from build123d import *

# Parameters (mm, degrees)
SKETCH_1_R          = 30
EXTRUDE_1_DEPTH     = 98
SKETCH_2_R          = 17.5
CUT_EXTRUDE_1_DEPTH = 25
SKETCH_3_R          = 12.5
CUT_EXTRUDE_2_DEPTH = 25


with BuildPart() as part:
    # 草图1 → 凸台-拉伸1 (new body)
    with BuildSketch(Plane.XY):
        with Locations((-39.098360656, 16.475409836)):
            Circle(SKETCH_1_R)
    extrude(amount=EXTRUDE_1_DEPTH)

    # 草图2 → 切除-拉伸1 (cut)
    with BuildSketch(Plane.XY.offset(98)):
        with Locations((-39.098360656, 16.475409836)):
            Circle(SKETCH_2_R)
    extrude(amount=-CUT_EXTRUDE_1_DEPTH, mode=Mode.SUBTRACT)

    # 草图3 → 切除-拉伸2 (cut)
    with BuildSketch(Plane(origin=(0, 0, 0), x_dir=(-1, 0, 0), z_dir=(0, 0, -1))):
        with Locations((39.098360656, 16.475409836)):
            Circle(SKETCH_3_R)
    extrude(amount=-CUT_EXTRUDE_2_DEPTH, mode=Mode.SUBTRACT)


solid = part.part
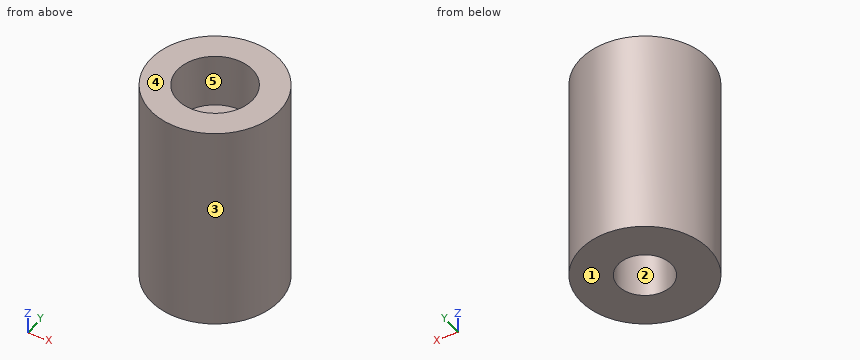
Model file for the job. Use its own axes, mm. Face numbers are marked on the shaded views. A direction names the side the tool comes from. Round coordinates to 2 decimals unless told otherwise and drop trailing zeros. Order: outer loops, then holes, each group sorted by start corner. A loop starts at its lowest first (then second) coordinate and runs counter-clockwise, first axis right, second up.
(1) Pin check, flat tips, straight feed: pin 1 (2 mm diameter, centred on x = -22, z = 37.5, fed in from +Y); pin 2 (2 mm diameter, centred on x = -32.5, y = 25.5, fed in from -Z); pin 3 (8 mm diameter, centred on y = -4, z = 80.5, fed in from -X). Stop position of each tip, or through.
(2) Band-saw the part on A-A (y = 23). List the corners of the cut face in (x, z), then the cut area to 3 significant figures.
(3) Band-saw the part on B-B (x = -44). List the corners of the cut face in (y, z), then the cut area to 3 significant figures.
(4) Pull direction Y, two halves, no side cores. Call the marked faces 3, 4 and 5: released by +Y, released by -Y, zero draft, split by the parting line, or undercut.
(5) Band-saw the part on D-D (z = 31). List the corners of the cut face in (x, y), then the cut area to 3 significant figures.
(6) Drill centre lines: line 1 (X direction, y = 17, z = 82.5); line 2 (Z direction, x = -45.5, y = 9.5); line 3 (Y direction, x = -44, z = 86). Where is each one in solid material? Low to high.
(7) 3-axis set-ups, long thin cutter, end or side, ignore diameter. For the marked faces 1 and 2: which of +Z, -Z, +X, -X, +Y, -Y reach the whole face in a straight line?
(8) Band-saw the part on C-C (z = 79.5). List the corners of the cut face in (x, y).
Verdict:
1. pin 1: stops at y = 41.79
1. pin 2: stops at z = 25
1. pin 3: stops at x = -64.17
2. outline: (-68.38, 0) - (-49.76, 0) - (-49.76, 25) - (-28.44, 25) - (-28.44, 0) - (-9.82, 0) - (-9.82, 98) - (-22.86, 98) - (-22.86, 73) - (-55.34, 73) - (-55.34, 98) - (-68.38, 98) - close
2. area: 4,390 mm2
3. outline: (-13.12, 0) - (4.98, 0) - (4.98, 25) - (27.97, 25) - (27.97, 0) - (46.07, 0) - (46.07, 98) - (33.27, 98) - (33.27, 73) - (-0.32, 73) - (-0.32, 98) - (-13.12, 98) - close
3. area: 4,390 mm2
4. face 3: split by the parting line
4. face 4: zero draft
4. face 5: undercut
5. outline: circle Ø60 at (-39.1, 16.48)
5. area: 2,830 mm2
6. line 1: x = -69.09 to -56.59, -21.61 to -9.1
6. line 2: z = 25 to 73
6. line 3: y = -13.12 to -0.32, 33.27 to 46.07
7. face 1: -Z, +X, -X, +Y, -Y
7. face 2: -Z
8. outline: circle Ø60 at (-39.1, 16.48); hole circle Ø35 at (-39.1, 16.48)
